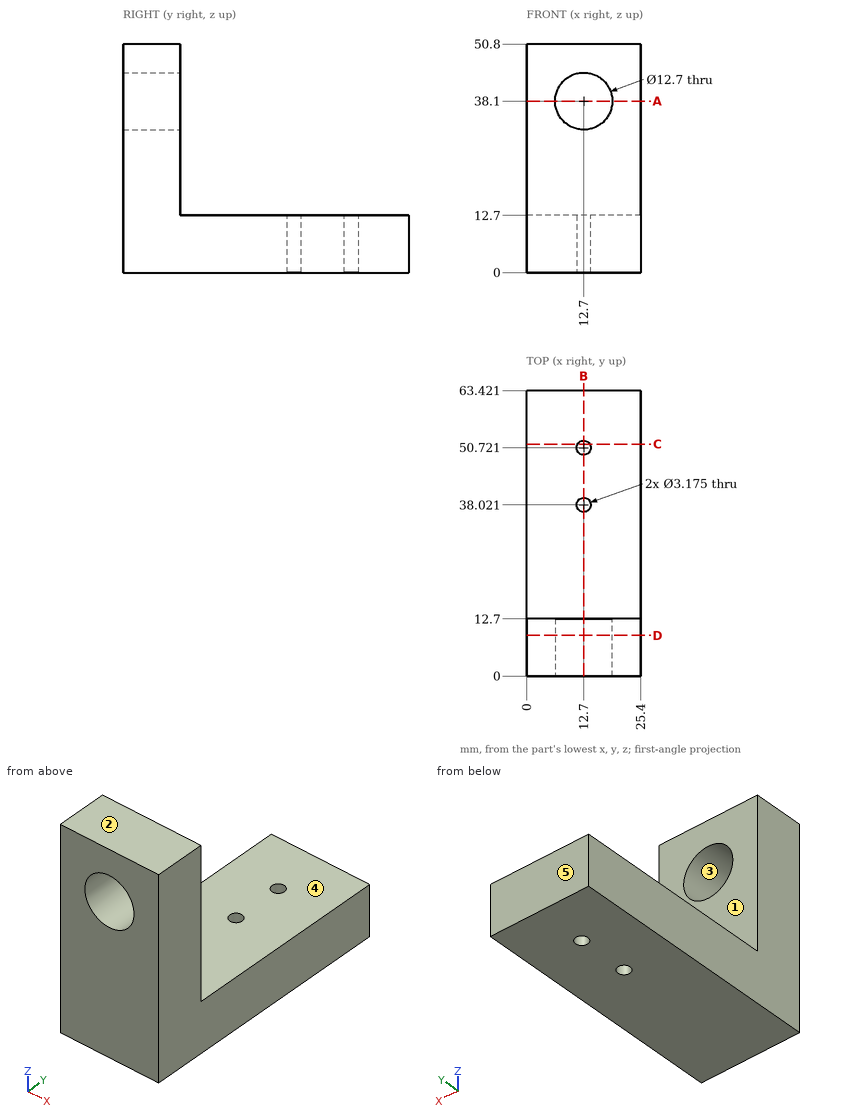
Could you check a few things on this drawing? It's one solid part, dimensions in mm from its lowest x, y, z. A direction names the side the tool comes from. Give positions to 0.01 mm unless a question says otherwise; leave off trailing zeros. Order: outer loops, then holes, each group sorted by start corner. A loop starts at its lowest first (then second) coordinate and runs counter-clockwise, first axis right, second up. Notation, with made-up numbers: (70, 10) - (121, 10) arc R10 cw to (121, 16) - close; hole circle Ø7 at (30.5, 66). An arc over 180 degrees is marked (long way). One line per item, written item: value. Start each with the question number.
1. For P1, Ø1, axis at x = 9, y = 28.5, coming from the +Z side; P2, Ø11.5, axis at x = 12.7, z = 38.1, coming from the +Y side, each with a flat end and sliding along its axis, tell me the tip position at first contact or that it passes through.
2. For the marked faces 1 and 2, which set-ups out of +Z, -Z, +X, -X, +Y, -Y let a thin tool reach every point of the face, with its end or its side?
3. Imagine slicing it at C-C on y = 51.5. List the corners of the cut face in (x, z) for me.
4. If I drill on probe 1 along Y at (x, z) = (12.7, 5.5); probe 2 along Z at (x, y) = (12.7, 5); probe 3 along Y at (x, z) = (11.5, 11.5), over which ranges is the centre line in solid material (lowest first)?
5. Imagine slicing it at D-D on y = 9. List the corners of the cut face in (x, z) for me, plus the area to 3 significant figures.
6. Imagine slicing it at B-B on x = 12.7. List the corners of the cut face in (y, z) for me.
7. Thinking about a two-plate mould opening in Z: for the marked faces 3, 4 and 5, which applies, +Z half, -Z half, draft (parallel to the pull), parting line (faces both ways), or undercut?
8. Imagine slicing it at A-A on z = 38.1. List the corners of the cut face in (x, y) for me, plus the area to 3 significant figures.
Values:
1. P1: z = 12.7
1. P2: through
2. face 1: +Z, +X, -X, +Y
2. face 2: +Z, +X, -X, +Y, -Y
3. outline: (0, 0) - (11.32, 0) - (11.32, 12.7) - (0, 12.7) - close; (14.08, 0) - (25.4, 0) - (25.4, 12.7) - (14.08, 12.7) - close
4. probe 1: 0 to 36.43, 39.61 to 49.13, 52.31 to 63.42
4. probe 2: 0 to 31.75, 44.45 to 50.8
4. probe 3: 0 to 36.98, 39.06 to 49.68, 51.76 to 63.42
5. outline: (0, 0) - (25.4, 0) - (25.4, 50.8) - (0, 50.8) - close; hole circle Ø12.7 at (12.7, 38.1)
5. area: 1,160 mm²
6. outline: (0, 0) - (36.43, 0) - (36.43, 12.7) - (12.7, 12.7) - (12.7, 31.75) - (0, 31.75) - close; (0, 44.45) - (12.7, 44.45) - (12.7, 50.8) - (0, 50.8) - close; (39.61, 0) - (49.13, 0) - (49.13, 12.7) - (39.61, 12.7) - close; (52.31, 0) - (63.42, 0) - (63.42, 12.7) - (52.31, 12.7) - close
7. face 3: undercut
7. face 4: +Z half
7. face 5: draft
8. outline: (0, 0) - (6.35, 0) - (6.35, 12.7) - (0, 12.7) - close; (19.05, 0) - (25.4, 0) - (25.4, 12.7) - (19.05, 12.7) - close
8. area: 161 mm²
